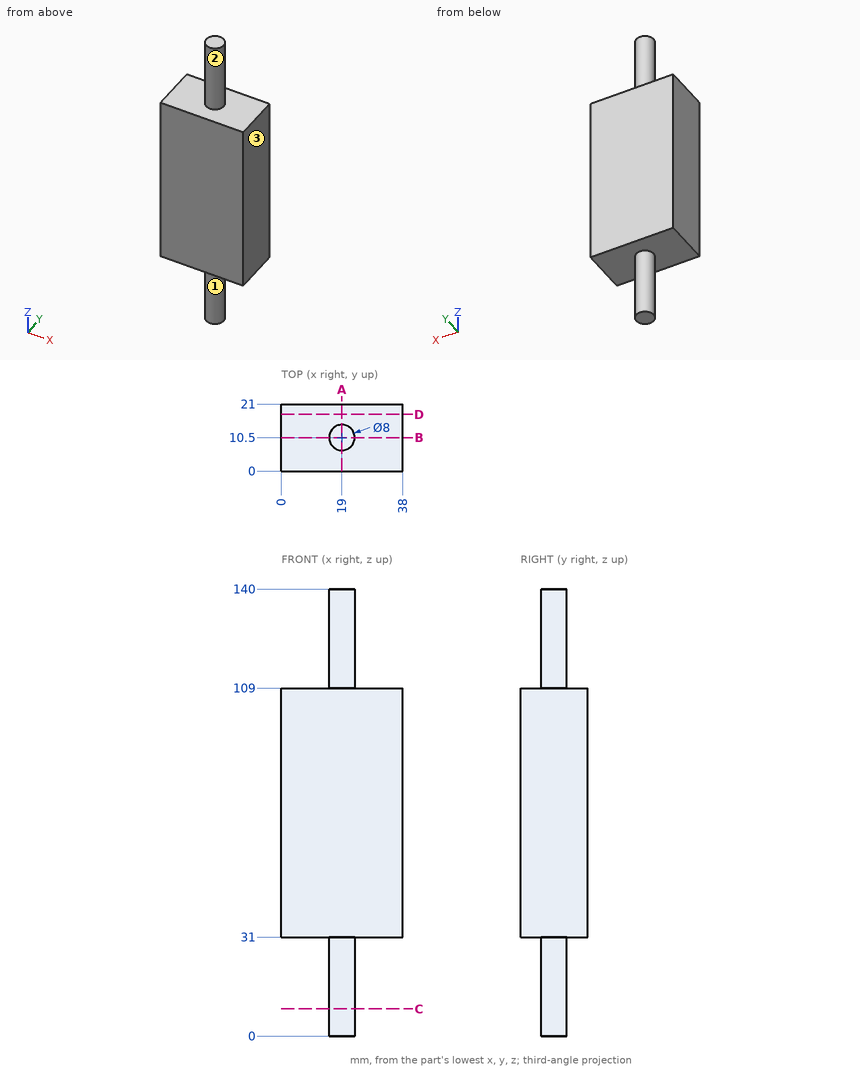
Verification items for this drawing (mm, ordinates from the low corner). A direction names the side the tool comes from. Give positions to 0.01 mm unless a question says otherwise; leave off trailing zeros. Write each loop counter-clockwise with the first axis right and the second up, starting at its lowest first coordinate (ties: lowest second). Pieces come first, ordered by that corner, then holes. Notation, with made-up numbers: (50.5, -15.75) - (92.5, -15.75) arc R23 ccw to (92.5, -5.75) - close; hole circle Ø5 at (26.5, -17). An arc over 180 degrees is marked (long way). Answer as CSV lines item,"result". Start each with the question number.
1. Thickness scan on line 1 (Z direction, x = 3.5, y = 18.25). Record the ranges inside material, lowest first.
2. Depth check by flat-ended pin: pin 1 (4 mm diameter, centred on x = 26, y = 8.5, fed in from +Z); pin 2 (6 mm diameter, centred on x = 31, y = 17, fed in from -Z). Enter the tip coordinate at first touch or a pass-through.
3. Sectioned sample at A-A (x = 19). Record the boundary of the cut face in (y, z), then the cut area to 3 significant figures.
4. Sectioned sample at C-C (z = 8.5). Record the boundary of the cut face in (x, y).
5. Set-up check for the marked faces 1, 2 and 3: record each of +Z, -Z, +X, -X, +Y, -Y from which the full face is reachable in a straight line by a thin tool's end or side.
6. Sectioned sample at B-B (y = 10.5). Record the boundary of the cut face in (x, z).
7. Sectioned sample at D-D (y = 17.75). Record the boundary of the cut face in (x, z).
Derived:
1,line 1,"31 to 109"
2,pin 1,"z = 109"
2,pin 2,"z = 31"
3,outline,"(0, 31) - (6.5, 31) - (6.5, 0) - (14.5, 0) - (14.5, 31) - (21, 31) - (21, 109) - (14.5, 109) - (14.5, 140) - (6.5, 140) - (6.5, 109) - (0, 109) - close"
3,area,"2,130 mm²"
4,outline,"circle Ø8 at (19, 10.5)"
5,face 1,"-Z"
5,face 2,"+Z"
5,face 3,"+Z, -Z, +X, +Y, -Y"
6,outline,"(0, 31) - (15, 31) - (15, 0) - (23, 0) - (23, 31) - (38, 31) - (38, 109) - (23, 109) - (23, 140) - (15, 140) - (15, 109) - (0, 109) - close"
7,outline,"(0, 31) - (38, 31) - (38, 109) - (0, 109) - close"
